Here's how the part is built. I have some questions about the finished solid (model axes, mm). Coordinates: 2 decimals unless noted, no trailing zeros. Order: outer loops, then holes, each group sorted by start corner. A loop starts at its lowest first (then second) coordinate and runs counter-clockwise, first axis right, second up. Notation, with made-up numbers: M 16.25,-2.5 L 26.25,-2.5 A18 cw 26.25,22.5 Z; hole C 78.25,33.5 d5. An arc over 180 degrees is marked long. One line per question, with ' | ' between items. Start each with the question number.
Autodesk Inventor part; units mm, degrees
ref_plane "YZ Plane" through (0, 0, 0) normal (1, 0, 0) x (0, 1, 0)
ref_plane "XZ Plane" through (0, 0, 0) normal (0, 1, 0) x (-1, 0, 0)
ref_plane "XY Plane" through (0, 0, 0) normal (0, 0, 1) x (1, 0, 0)
sketch "Sketch1" plane through (0, 0, 0) normal (0, 1, 0) x (-1, 0, 0)
  line L0 (32, 55) -> (-32, 55)
  line L1 (-32, 55) -> (-32, -55)
  line L2 (-32, -55) -> (32, -55)
  line L3 (32, -55) -> (32, 55)
  line L4 (32, 55) -> (-32, -55) construction
  line L5 (-32, 55) -> (32, -55) construction
  circle A0 centre (32, 55) radius 4.2425
  circle A1 centre (32, -55) radius 4.2425
  circle A2 centre (-32, 55) radius 4.2425
  circle A3 centre (-32, -55) radius 4.2425
  point P0 (0, 0)
  dimension "d0" = 64
  dimension "d1" = 110
  dimension "d2" = 8.485
  dimension "d5" = 110
  dimension "d8" = 64
extrude "Extrusion1" add sketch "Sketch1" along normal blind 3
sketch "Sketch2" plane through (0, 3, 0) normal (0, 1, 0) x (1, 0, 0)
  line L0 (32, -50.7575) -> (32, 50.7575)
  arc A0 (32, 50.7575) -> (27.7575, 55) centre (32, 55) ccw
  line L1 (27.7575, 55) -> (-27.7575, 55)
  arc A1 (-27.7575, 55) -> (-32, 50.7575) centre (-32, 55) ccw
  line L2 (-32, 50.7575) -> (-32, -50.7575)
  arc A2 (-32, -50.7575) -> (-27.7575, -55) centre (-32, -55) ccw
  line L3 (-27.7575, -55) -> (27.7575, -55)
  arc A3 (27.7575, -55) -> (32, -50.7575) centre (32, -55) ccw
  circle A4 centre (-32, -55) radius 2.15
  circle A5 centre (-32, 55) radius 2.15
  circle A6 centre (32, -55) radius 2.15
  circle A7 centre (32, 55) radius 2.15
  point P0 (0, 0)
  dimension "d13" = 4.3
  dimension "d16" = 110
  dimension "d19" = 64
extrude "Extrusion2" cut sketch "Sketch2" against normal blind 3 contours A4 | A5 | A6 | A7
sketch "Sketch3" plane through (0, 3, 0) normal (0, 1, 0) x (1, 0, 0)
  line L0 (-8, -39.3) -> (8, -39.3)
  line L1 (8, -39.3) -> (8, -7.8)
  line L2 (8, -7.8) -> (-8, -7.8)
  line L3 (-8, -7.8) -> (-8, -39.3)
  line L4 (-32, 50.7575) -> (-32, -50.7575)
  line L5 (32, -50.7575) -> (32, 50.7575)
  line L6 (-27.7575, -55) -> (27.7575, -55)
  point P0 (0, 0)
  dimension "d24" = 16
  dimension "d25" = 31.5
  dimension "d26" = 24
  dimension "d27" = 24
  dimension "d28" = 15.7
extrude "Extrusion3" cut sketch "Sketch3" against normal blind 3
sketch "Sketch4" plane through (0, 3, 0) normal (0, 1, 0) x (1, 0, 0)
  circle A0 centre (0, 7.9) radius 3.4
  line L0 (0, 82.9395) -> (0, -82.9395)
  circle A1 centre (0, 23.6) radius 3.4
  circle A2 centre (0, 39.3) radius 3.4
  line L1 (27.7575, 55) -> (-27.7575, 55)
  line L2 (-8, -7.8) -> (8, -7.8)
  point P0 (0, 0)
  dimension "d31" = 6.8
  dimension "d32" = 6.8
  dimension "d33" = 6.8
  dimension "d34" = 15.7
  dimension "d35" = 15.7
  dimension "d36" = 15.7
  dimension "d37" = 15.7
extrude "Extrusion4" cut sketch "Sketch4" against normal blind 3
sketch "Sketch5" plane through (0, 3, 0) normal (0, 1, 0) x (1, 0, 0)
  circle A0 centre (0, 23.6) radius 3.4
  circle A1 centre (0, 7.9) radius 3.4
  circle A2 centre (0, 39.3) radius 3.4
  line L0 (8, -7.8) -> (8, -39.3)
  line L1 (8, -39.3) -> (-8, -39.3)
  line L2 (-8, -39.3) -> (-8, -7.8)
  line L3 (-8, -7.8) -> (8, -7.8)
  circle A3 centre (32, -55) radius 2.15
  circle A4 centre (-32, -55) radius 2.15
  circle A5 centre (-32, 55) radius 2.15
  circle A6 centre (32, 55) radius 2.15
  line L4 (32, -50.7575) -> (32, 50.7575)
  arc A7 (32, 50.7575) -> (27.7575, 55) centre (32, 55) ccw
  line L5 (27.7575, 55) -> (-27.7575, 55)
  arc A8 (-27.7575, 55) -> (-32, 50.7575) centre (-32, 55) ccw
  line L6 (-32, 50.7575) -> (-32, -50.7575)
  arc A9 (-32, -50.7575) -> (-27.7575, -55) centre (-32, -55) ccw
  line L7 (-27.7575, -55) -> (27.7575, -55)
  arc A10 (27.7575, -55) -> (32, -50.7575) centre (32, -55) ccw
  circle A11 centre (-32, -55) radius 2.15
  circle A12 centre (-32, -55) radius 4.2425
  circle A13 centre (-32, 55) radius 4.2425
  circle A14 centre (32, -55) radius 4.2425
  circle A15 centre (32, 55) radius 4.2425
  line L8 (-32, -50.7575) -> (-32, 50.7575)
  line L9 (-27.7575, 55) -> (27.7575, 55)
  line L10 (32, -50.7575) -> (32, 50.7575)
  line L11 (32, 50.7575) -> (32, -50.7575)
  line L12 (-27.7575, -55) -> (27.7575, -55)
  line L13 (27.7575, -55) -> (-27.7575, -55)
  point P0 (0, 0)
  dimension "d42" = 110
  dimension "d45" = 64
extrude "Extrusion5" add sketch "Sketch5" along normal blind 1.5 contours A14 L7 A12 L6 A13 L5 A15 L4
chamfer "Chamfer1" distance 1.5 angle 45 4 edges at (-32, 4.5, 0) (0, 4.5, 55) (32, 4.5, 0) (0, 4.5, -55)
equation "\"d26\" = d27"
equation "\"d32\" = d31"
equation "\"d33\" = d31"
equation "\"d34\" = d37"
equation "\"d35\" = d34"
equation "\"d36\" = d34"
properties part number "gora"
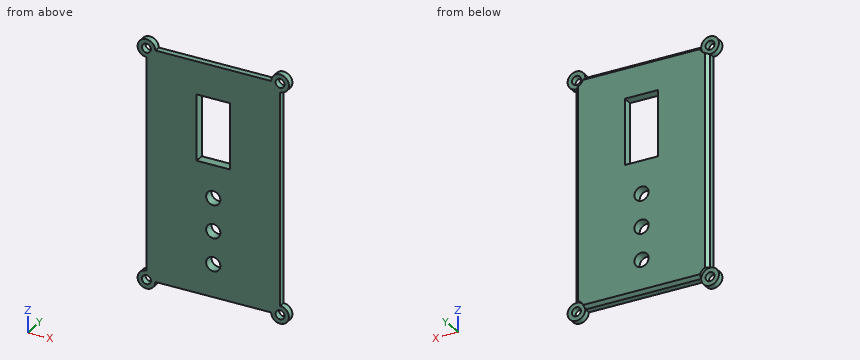
1. Imagine slicing it at C-C (x = 10). List the corners of the cut face in (y, z) for me.
2. I need wall thicknesses on line 1 (Z direction, x = 0, y = 2.15); line 2 (X direction, y = 1.4, z = 35); line 3 (Z direction, x = 6, y = 0.85). Which ranges of each line are inside material? Lowest first, please.
3. Imagine slicing it at B-B (x = -6). List the corners of the cut face in (y, z) for me.
4. Will these pins go through, and if not, where does the flat tip stop? pin 1 (7 mm diameter, centred on x = -33, z = 55, fed in from +Y); pin 2 (1.3 mm diameter, centred on y = 2, z = 27.5, fed in from +X); pin 3 (1 mm diameter, centred on y = 2, z = 15, fed in from -X).
5. Imagine slicing it at A-A (z = -7.9). List the corners of the cut face in (x, y) for me, then the cut area to 3 significant figures.
Entries:
1) outline: M 0,-55 L 3,-55 L 4.5,-53.5 L 4.5,53.5 L 3,55 L 0,55 Z
2) line 1: -55 to -42.7, -35.9 to -27, -20.2 to -11.3, -4.5 to 7.8, 39.3 to 55 | line 2: -32 to -8, 8 to 32 | line 3: -55 to 7.8, 39.3 to 55
3) outline: M 0,-55 L 3,-55 L 4.5,-53.5 L 4.5,7.8 L 0,7.8 Z; M 0,39.3 L 4.5,39.3 L 4.5,53.5 L 3,55 L 0,55 Z
4) pin 1: y = 3 | pin 2: x = 32 | pin 3: x = -32
5) outline: M -32,0 L -3.4,0 L -3.4,4.5 L -30.5,4.5 L -32,3 Z; M 3.4,0 L 32,0 L 32,3 L 30.5,4.5 L 3.4,4.5 Z | area: 255 mm²
